```python
from build123d import *

# Parameters (mm, degrees)
SKETCH1_R           = 6.25
SKETCH1_R_2         = 2.6
SKETCH1_R_3         = 6
SKETCH1_W           = 7.5
SKETCH1_H           = 50.316251501
BOSS_EXTRUDE1_DEPTH = 11.5
FILLET1_R           = 10
SKETCH2_W           = 12.5
SKETCH2_H           = 36.489359976
CUT_EXTRUDE1_DEPTH  = 5
FILLET2_R           = 10


with BuildPart() as part:
    # Sketch1 → Boss-Extrude1 (new body)
    # profile 1 of 3: a face of its own
    with BuildSketch(Plane(origin=(0, 0, 0), x_dir=(1, 0, 0), z_dir=(0, 1, 0))):
        with Locations((0, 60)):
            Circle(SKETCH1_R)
        with Locations(Location((0, 60, 0), (0, 0, 270))):
            Circle(SKETCH1_R_2, mode=Mode.SUBTRACT)
    # profile 2 of 3: a face of its own
    with BuildSketch(Plane(origin=(0, 0, 0), x_dir=(1, 0, 0), z_dir=(0, 1, 0))):
        Circle(SKETCH1_R_3)
        with Locations(Location((0, 0, 0), (0, 0, 270))):
            Circle(SKETCH1_R_2, mode=Mode.SUBTRACT)
    # profile 3 of 3: a face of its own
    with BuildSketch(Plane(origin=(0, 0, 0), x_dir=(1, 0, 0), z_dir=(0, 1, 0))):
        with Locations((0, 29.84187425)):
            Rectangle(SKETCH1_W, SKETCH1_H)
    extrude(amount=BOSS_EXTRUDE1_DEPTH)

    # Fillet1
    fillet1_edges = [part.edges().sort_by_distance(p)[0] for p in [
        (-3.75, 5.75, -55),
        (3.75, 5.75, -55),
        (3.75, 5.75, -4.683748499),
        (-3.75, 5.75, -4.683748499),
    ]]
    fillet(fillet1_edges, radius=FILLET1_R)

    # Sketch2 → Cut-Extrude1 (cut)
    with BuildSketch(Plane.XZ):
        with Locations((0, -48.005320012)):
            Rectangle(SKETCH2_W, SKETCH2_H)
    extrude(amount=-CUT_EXTRUDE1_DEPTH, mode=Mode.SUBTRACT)

    # Fillet2
    # the kernel refuses this fillet: 10 mm, written as the material it adds along each edge
    with BuildSketch(Plane(origin=(-3.75, 5, -29.760640024), x_dir=(0, -1, 0), z_dir=(1, 0, 0))) as fillet2_piece_1:
        with BuildLine():
            CenterArc((10, 8.660254038), FILLET2_R, 180, 60)
            Line((0, 8.660254038), (-0.2, 8.660254038))
            Line((-0.2, 8.660254038), (-0.2, 0))
            Line((-0.2, 0), (0, -0.2))
            ThreePointArc((0, -0.2), (2.5, -0.2), (4.9, -0.173205081))
            Line((4.9, -0.173205081), (5, 0))
        make_face()
    extrude(amount=7.5)


solid = part.part
```
Input: part model. Units: mm. Frame: model coordinates. A direction names the side the tool comes from. Give positions to 0.01 mm unless a question says otherwise; leave off trailing zeros. Order: outer loops, then holes, each group sorted by start corner. A loop starts at its lowest first (then second) coordinate and runs counter-clockwise, first axis right, second up. Notation, with made-up numbers: M -38,68 L -31,68 A26 ccw -31,91 Z; hole C -20.5,26 d2. An arc over 180 degrees is marked long. Return JSON: item names as keys, results as strings.
Item 1: Cut plane A-A (z = -60). Return loops of the section in (x, y).
Solutions:
{"outline": "M -6.25,5 L -2.6,5 L -2.6,11.5 L -6.25,11.5 Z; M 2.6,5 L 6.25,5 L 6.25,11.5 L 2.6,11.5 Z"}
Item 2: Cut plane C-C (y = 10.5). Return loops of the section in (x, z).
Solutions:
{"outline": "M -5.29,-56.67 A6.25 ccw long 5.29,-56.67 A10 cw 3.75,-51.34 L 3.75,-8.18 A10 cw 5.16,-3.07 A6 ccw long -5.16,-3.07 A10 cw -3.75,-8.18 L -3.75,-51.34 A10 cw Z; hole C 0,-60 d5.2; hole C 0,0 d5.2"}
Item 3: Ray query, probe 1 along Z at (x, y) = (-1, 8.75); probe 2 along Z at (x, y) = (-0.75, 10.75); probe 3 along X at (y, z) = (9.25, 0). Return the intervals inside material, ascending.
Solutions:
{"probe 1": "-66.17 to -62.4, -57.6 to -2.4, 2.4 to 5.92", "probe 2": "-66.2 to -62.49, -57.51 to -2.49, 2.49 to 5.95", "probe 3": "-6 to -2.6, 2.6 to 6"}
Item 4: Pull-direction query (Z, two-part tool) for faces 1 (the cylindrical face through (-4.131, 8.296, -54.075)), 2 (the flat face through (0, 11.5, -31)), 3 (the cylindrical face through (-0.053, 3.697, -33.485)); classes: +Z half, -Z half, draft (parallel to the pull), parting line (faces both ways), or undercut.
Solutions:
{"face 1": "undercut", "face 2": "draft", "face 3": "-Z half"}
Item 5: Access query for faces 4 (the cylindrical face through (0.1, 8.2, -62.6)), 5 (the cylindrical face through (4.131, 8.296, -54.075)), 6 (the flat face through (-3.75, 7, -25)), 7 (the flat face through (0, 5, -52)). Directions: +Z, -Z, +X, -X, +Y, -Y. A direction counts if a zero-diameter tool reaches every point of the face in a straight line with its end or side. Return the directions, or none.
Solutions:
{"face 4": "+Y, -Y", "face 5": "+X, +Y, -Y", "face 6": "-X, +Y, -Y", "face 7": "-Z, +X, -X, -Y"}
Item 6: First-contact query: P1, Ø1.5, axis at y = 8, z = -9, coming from the -X side; P2, Ø1, axis at y = 4.5, z = -6.5, coming from the +X side. Flat tips, straight axial feed; report the tip coordinate or a pass-through.
Solutions:
{"P1": "x = -3.75", "P2": "x = 3.99"}
Item 7: Cut plane B-B (x = 0). Return loops of the section in (y, z).
Solutions:
{"outline": "M 0,-29.76 A10 cw 5,-38.42 L 5,-57.4 L 11.5,-57.4 L 11.5,-2.6 L 0,-2.6 Z; M 0,2.6 L 11.5,2.6 L 11.5,6 L 0,6 Z; M 5,-66.25 L 11.5,-66.25 L 11.5,-62.6 L 5,-62.6 Z"}
Item 8: Cut plane D-D (z = 0). Return loops of the section in (x, y).
Solutions:
{"outline": "M -6,0 L -2.6,0 L -2.6,11.5 L -6,11.5 Z; M 2.6,0 L 6,0 L 6,11.5 L 2.6,11.5 Z"}
